Geometry: final body of the model. Coordinates: model frame, mm. Face numbers are marked on the shaded views. Coordinates: 2 decimals unless noted, no trailing zeros. One line per item, written item: value. Start each with the question number.
Item 1: Mould query, pull axis Y, two halves, no side actions, for the marked faces 1, 2, 3 and 4. Classes: +Y half, -Y half, draft (parallel to the pull), parting line (faces both ways), or undercut.
Item 2: Ray query, probe 1 along X at (y, z) = (8.25, 1); probe 2 along Y at (x, z) = (-27, 1); probe 3 along X at (y, z) = (5.25, 8). Return the intervals inside material, ascending. Write a range as from..to.
Item 3: Contact query for flat-ended pins moving along their axis: pin 1 Ø3 at (x, y) = (19, 2) entering from -Z; pin 2 Ø1.5 at (y, z) = (9.5, -15.5) entering from -X. Output: stop coordinate, or through.
Item 4: Section query A-A on y = 4.25. Give the number of separate pieces and of enclosed holes in the cut face, then the cut area to 3 significant figures.
from build123d import *

# Parameters (mm, degrees)
BOSS_EXTRUDE1_DEPTH = 15
SKETCH2_R           = 5
CUT_EXTRUDE1_DEPTH  = 41
FILLET1_R           = 7
SKETCH3_R           = 8
CUT_EXTRUDE2_DEPTH  = 16
CHAMFER1_SIZE       = 1


with BuildPart() as part:
    # Sketch1 → Boss-Extrude1 (new body)
    with BuildSketch(Plane(origin=(0, 0, 0), x_dir=(1, 0, 0), z_dir=(0, 1, 0))):
        with BuildLine():
            Line((15.5, -20), (-34.5, -20))
            Line((-34.5, -20), (-34.5, 20))
            Line((-34.5, 20), (15.5, 20))
            ThreePointArc((15.5, 20), (28.935028843, 14.435028843), (34.5, 1))
            Line((34.5, 1), (34.5, -1))
            ThreePointArc((34.5, -1), (28.935028843, -14.435028843), (15.5, -20))
        make_face()
    extrude(amount=BOSS_EXTRUDE1_DEPTH)

    # Sketch2 → Cut-Extrude1 (cut, through all)
    with BuildSketch(Plane.XY.offset(20)):
        with Locations((-27, 7.5)):
            Circle(SKETCH2_R)
    extrude(amount=-CUT_EXTRUDE1_DEPTH, mode=Mode.SUBTRACT)

    # Fillet1
    fillet1_edges = [part.edges().sort_by_distance(p)[0] for p in [
        (-34.5, 15, 0),
        (-34.5, 0, 0),
    ]]
    fillet(fillet1_edges, radius=FILLET1_R)

    # Sketch3 → Cut-Extrude2 (cut, through all)
    with BuildSketch(Plane(origin=(0, 15, 0), x_dir=(1, 0, 0), z_dir=(0, 1, 0))):
        with Locations((15.5, -1)):
            Circle(SKETCH3_R)
    extrude(amount=-CUT_EXTRUDE2_DEPTH, mode=Mode.SUBTRACT)

    # Chamfer1
    chamfer1_edges = [part.edges().sort_by_distance(p)[0] for p in [
        (28.935028843, 15, 14.435028843),
        (34.5, 15, 0),
        (28.935028843, 15, -14.435028843),
        (-6, 15, -20),
        (-34.5, 7.5, 20),
        (-34.5, 7.5, -20),
        (-6, 0, 20),
        (-6, 15, 20),
        (-32.449747468, 12.949747468, 20),
        (-32.449747468, 2.050252532, 20),
        (-32.449747468, 12.949747468, -20),
        (-32.449747468, 2.050252532, -20),
        (7.5, 0, 1),
        (7.5, 15, 1),
        (-6, 0, -20),
        (28.935028843, 0, -14.435028843),
        (34.5, 0, 0),
        (28.935028843, 0, 14.435028843),
    ]]
    chamfer(chamfer1_edges, length=CHAMFER1_SIZE)


solid = part.part
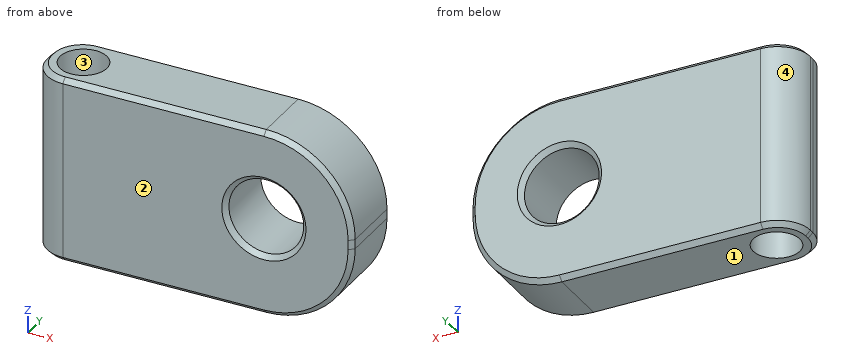
Reply:
1. face 1: draft
1. face 2: -Y half
1. face 3: undercut
1. face 4: +Y half
2. probe 1: x = -34.5..-31.94, -22.06..7.5, 23.5..34.5
2. probe 2: y = 0..2.5, 12.5..15
2. probe 3: x = -34.28..-31.47, -22.53..11.63, 19.37..33.16
3. pin 1: stops at z = -19.89
3. pin 2: stops at x = -34.46
4. separate pieces: 2
4. enclosed holes: 1
4. area: 2,080 mm²
